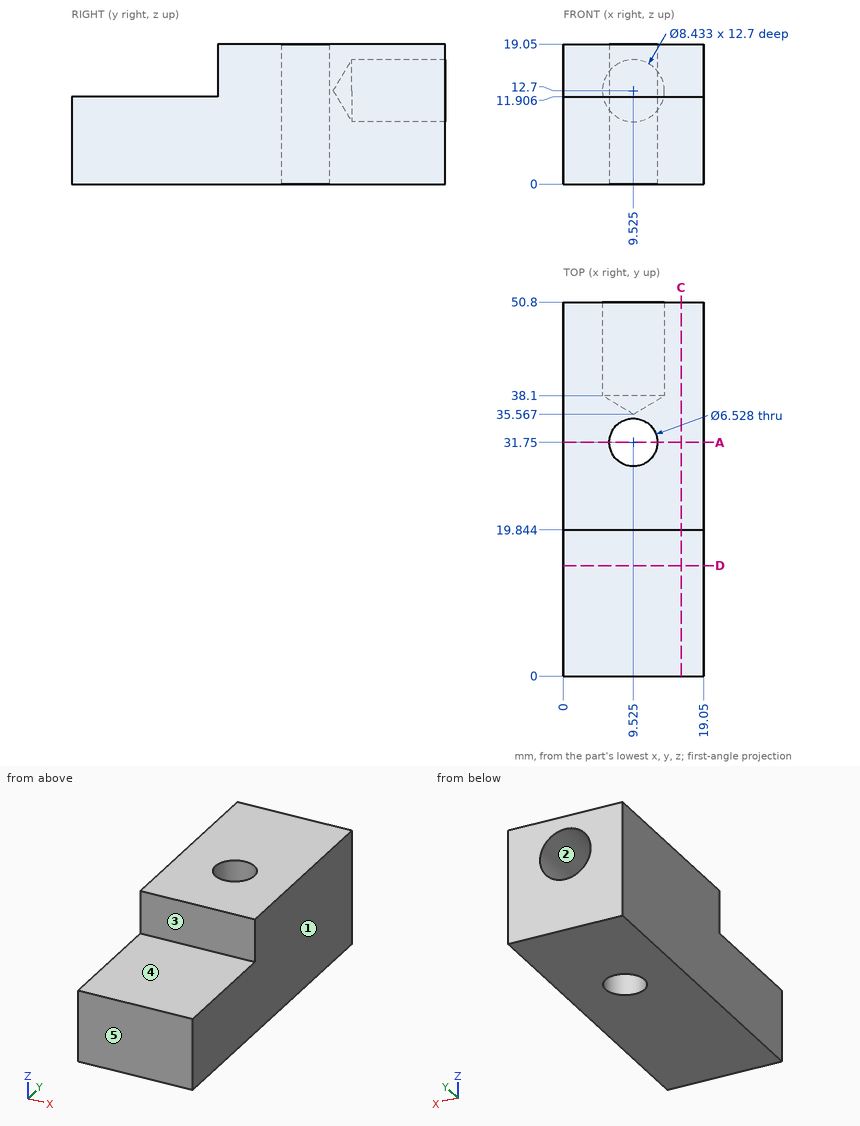
Geometry: see drawing. Coordinates: mm, zero at the bounding-box minimum. A direction names the side the tool comes from. Give positions to 0.01 mm unless a question says otherwise; leave off trailing zeros. Write each loop counter-clockwise with the first axis right and the second up, starting at its lowest first coordinate (ties: lowest second). Pieces come first, ordered by that corner, then holes. Notation, with made-up numbers: M -20,-25 L 29,-25 A17 cw 29,-14 Z; hole C 87.5,-3 d4. An arc over 180 degrees is marked long. Answer in a Markdown table with one row per item. Add a question column.
(1) Ray query, line 1 (X direction, y = 44.75, z = 12.7); line 2 (Z direction, x = 9.5, y = 46.5); line 3 (Y direction, x = 4.75, z = 13). Return the intervals inside material, ascending.
(2) Reachability of the marked faces 4 and 5 from +Z, -Z, +X, -X, +Y, -Y: full face, straight path, thin tool, end or side. Return the list, or none.
(3) Section A-A on y = 31.75. Return loops of the section in (x, z).
(4) Section D-D on y = 15. Return loops of the section in (x, z).
(5) Mould query, pull axis X, two halves, no side actions, for the marked faces 1, 2 and 3. Classes: +X half, -X half, draft (parallel to the pull), parting line (faces both ways), or undercut.
(6) First-contact query: pin 1 (5.5 mm diameter, centred on x = 11, y = 10.5, fed in from +Z); pin 2 (2 mm diameter, centred on x = 10, z = 17, fed in from -Y). Flat tips, straight axial feed; report the tip coordinate or a pass-through.
(7) Section C-C on x = 16. Return loops of the section in (y, z), and give its area (3 significant figures).
Result set:
| question | item | result |
|---|---|---|
| 1 | line 1 | x = 0 to 5.31, 13.74 to 19.05 |
| 1 | line 2 | z = 0 to 8.48, 16.92 to 19.05 |
| 1 | line 3 | y = 19.84 to 50.8 |
| 2 | face 4 | +Z, +X, -X, -Y |
| 2 | face 5 | +Z, -Z, +X, -X, -Y |
| 3 | outline | M 0,0 L 6.26,0 L 6.26,19.05 L 0,19.05 Z; M 12.79,0 L 19.05,0 L 19.05,19.05 L 12.79,19.05 Z |
| 4 | outline | M 0,0 L 19.05,0 L 19.05,11.91 L 0,11.91 Z |
| 5 | face 1 | +X half |
| 5 | face 2 | undercut |
| 5 | face 3 | draft |
| 6 | pin 1 | stops at z = 11.91 |
| 6 | pin 2 | stops at y = 19.84 |
| 7 | outline | M 0,0 L 50.8,0 L 50.8,19.05 L 19.84,19.05 L 19.84,11.91 L 0,11.91 Z |
| 7 | area | 826 mm^2 |
